from build123d import *

# Parameters (mm, degrees)
SCHIZZO1_R                        = 31.2
SCHIZZO1_R_2                      = 22.5
ESTRUSIONE_ESTRUSIONE1_DEPTH      = 40
SCHIZZO2_R                        = 2.25
TAGLIO_ESTRUSIONE1_DEPTH          = 60.555688225
RIPETIZIONECIRCOLARE1_COUNT       = 9
SCHIZZO3_W                        = 40
SCHIZZO3_H                        = 62.4
TAGLIO_ESTRUSIONE2_DEPTH          = 39
ESTRUSIONE_ESTRUSIONE2_START      = -10
ESTRUSIONE_ESTRUSIONE2_DEPTH      = 10
SCHIZZO5_R                        = 8.05
TAGLIO_ESTRUSIONE3_DEPTH          = 5
SCHIZZO6_R                        = 6.05
TAGLIO_ESTRUSIONE6_DEPTH          = 57.31944602
SCHIZZO7_R                        = 3.75
TAGLIO_ESTRUSIONE7_DEPTH          = 5
RIPETIZIONECIRCOLARE2_COUNT       = 9
ESTRUSIONE_ESTRUSIONE3_DEPTH      = 2
ESTRUSIONE_ESTRUSIONE3_DEPTH_BACK = 5
SMUSSO1_SIZE                      = 2
RACCORDO2_R                       = 4
ESTRUSIONE_ESTRUSIONE4_DEPTH      = 40
ESTRUSIONE_ESTRUSIONE5_START      = -10
ESTRUSIONE_ESTRUSIONE5_DEPTH      = 10


# Some blends are built 0.0001 mm under size
with BuildPart() as part:
    # Schizzo1 → Estrusione-Estrusione1 (new body)
    with BuildSketch(Plane.XY):
        Circle(SCHIZZO1_R)
        Circle(SCHIZZO1_R_2, mode=Mode.SUBTRACT)
    extrude(amount=ESTRUSIONE_ESTRUSIONE1_DEPTH)

    # Schizzo2 → Taglio-Estrusione1 (cut, through all)
    with BuildSketch(Plane.XY.offset(40)):
        with Locations((0, 27)):
            Circle(SCHIZZO2_R)
    taglio_estrusione1 = extrude(amount=-TAGLIO_ESTRUSIONE1_DEPTH, mode=Mode.SUBTRACT)

    # RipetizioneCircolare1: Taglio-Estrusione1 ×9 about axis
    ripetizionecircolare1_axis = Axis((0, 0, 0), (0, 0, 1))
    for i in range(1, RIPETIZIONECIRCOLARE1_COUNT):
        add(taglio_estrusione1.rotate(ripetizionecircolare1_axis, i * 360 / RIPETIZIONECIRCOLARE1_COUNT), mode=Mode.SUBTRACT)

    # Schizzo3 → Taglio-Estrusione2 (cut)
    with BuildSketch(Plane(origin=(0, 0, 0), x_dir=(0, 0, -1), z_dir=(1, 0, 0))):
        with Locations((-20, 0)):
            Rectangle(SCHIZZO3_W, SCHIZZO3_H)
    extrude(amount=-TAGLIO_ESTRUSIONE2_DEPTH, mode=Mode.SUBTRACT)

    # Schizzo4 → Estrusione-Estrusione2 (add)
    with BuildSketch(Plane.XY.offset(40).offset(ESTRUSIONE_ESTRUSIONE2_START)):
        with BuildLine():
            Line((0, 22.5), (0, -22.5))
            ThreePointArc((0, -22.5), (22.5, 0), (0, 22.5))
        make_face()
        with BuildLine():
            ThreePointArc((22.5, 0), (15.909902577, 15.909902577), (0, 22.5))
            Line((0, 22.5), (0, -22.5))
            ThreePointArc((0, -22.5), (15.909902577, -15.909902577), (22.5, 0))
        make_face()
        with BuildLine():
            Line((0, -22.5), (0, 22.5))
            ThreePointArc((0, 22.5), (-22.5, 0), (0, -22.5))
        make_face()
    extrude(amount=ESTRUSIONE_ESTRUSIONE2_DEPTH)

    # Schizzo5 → Taglio-Estrusione3 (cut)
    with BuildSketch(Plane.XY.offset(40)):
        Circle(SCHIZZO5_R)
    extrude(amount=-TAGLIO_ESTRUSIONE3_DEPTH, mode=Mode.SUBTRACT)

    # Schizzo6 → Taglio-Estrusione6 (cut, through all)
    with BuildSketch(Plane.XY.offset(35)):
        Circle(SCHIZZO6_R)
    extrude(amount=-TAGLIO_ESTRUSIONE6_DEPTH, mode=Mode.SUBTRACT)

    # Schizzo7 → Taglio-Estrusione7 (cut)
    with BuildSketch(Plane.XY.offset(40)):
        with Locations((17.355265462, 20.683199964)):
            Circle(SCHIZZO7_R)
    taglio_estrusione7 = extrude(amount=-TAGLIO_ESTRUSIONE7_DEPTH, mode=Mode.SUBTRACT)

    # RipetizioneCircolare2: Taglio-Estrusione7 ×9 about axis
    ripetizionecircolare2_axis = Axis((0, 0, 0), (0, 0, 1))
    for i in range(1, RIPETIZIONECIRCOLARE2_COUNT):
        add(taglio_estrusione7.rotate(ripetizionecircolare2_axis, i * 360 / RIPETIZIONECIRCOLARE2_COUNT), mode=Mode.SUBTRACT)

    # Schizzo8 → Estrusione-Estrusione3 (add, two sides: drawn at the far end of the back side and taken through both)
    with BuildSketch(Plane(origin=(0, 0, 0), x_dir=(-1, 0, 0), z_dir=(0, 0, -1)).offset(-ESTRUSIONE_ESTRUSIONE3_DEPTH_BACK)):
        with BuildLine():
            Line((0, 31.2), (0, 33.2))
            ThreePointArc((0, 33.2), (-33.2, 0), (0, -33.2))
            Line((0, -33.2), (0, -31.2))
            ThreePointArc((0, -31.2), (-31.2, 0), (0, 31.2))
        make_face()
    extrude(amount=ESTRUSIONE_ESTRUSIONE3_DEPTH + ESTRUSIONE_ESTRUSIONE3_DEPTH_BACK)

    # Smusso1
    smusso1_edges = [part.edges().sort_by_distance(p)[0] for p in [
        (31.2, 0, 5),
    ]]
    chamfer(smusso1_edges, length=SMUSSO1_SIZE - 0.0001)  # a hair under: the kernel refuses the full size

    # Raccordo2
    # the kernel refuses this fillet: 4 mm, written as the material it adds along each edge
    with BuildSketch(Plane(origin=(0, 0, 30), x_dir=(0, -1, 0), z_dir=(-1, 0, 0))) as raccordo2_piece_1:
        with BuildLine():
            CenterArc((22.5 - RACCORDO2_R, -RACCORDO2_R), RACCORDO2_R, 0, 90)
            Line((22.5 - RACCORDO2_R, 0), (22.5, 0))
            Line((22.5, 0), (22.5, -RACCORDO2_R))
        make_face()
    revolve(axis=Axis((0, 0, 30), (0, 0, 1)), revolution_arc=180)

    # Schizzo9 → Estrusione-Estrusione4 (add)
    with BuildSketch(Plane.XY.offset(40)):
        with BuildLine():
            Line((0, 30.75), (0, 23.25))
            ThreePointArc((0, 23.25), (3.75, 27), (0, 30.75))
        make_face()
    extrude(amount=-ESTRUSIONE_ESTRUSIONE4_DEPTH)

    # Schizzo10 → Estrusione-Estrusione5 (add)
    with BuildSketch(Plane.XY.offset(40).offset(ESTRUSIONE_ESTRUSIONE5_START)):
        with BuildLine():
            Line((0, 22.5), (0, 31.2))
            Line((0, 31.2), (-15.587436356, 16.225961538))
            ThreePointArc((-15.587436356, 16.225961538), (-8.40136493, 20.872639203), (0, 22.5))
        make_face()
        with BuildLine():
            ThreePointArc((0, -22.5), (-8.40136493, -20.872639203), (-15.587436356, -16.225961538))
            Line((-15.587436356, -16.225961538), (0, -31.2))
            Line((0, -31.2), (0, -22.5))
        make_face()
    extrude(amount=ESTRUSIONE_ESTRUSIONE5_DEPTH)


solid = part.part
The model under review builds one solid part; all positions refer to its coordinate system, in mm. A direction names the side the tool comes from. Give positions to 0.01 mm unless a question says otherwise; leave off trailing zeros. Write each loop counter-clockwise with the first axis right and the second up, starting at its lowest first coordinate (ties: lowest second). Pieces come first, ordered by that corner, then holes. Notation, with made-up numbers: M 12,66.5 L 21,66.5 A13 cw 21,79.5 Z; hole C -0.5,24.5 d5. An arc over 180 degrees is marked long. One line per question, with ' | ' between items. Start each with the question number.
Item 1: For faces 4 (the flat face through (0, 28, 14)), 5 (the cylindrical face through (23.61, 2.41, 37.53)), 6 (the cylindrical face through (24.342, 4.787, 17.745)), 7 (the flat face through (24, 0, 0)), list the 3-axis set-ups (+Z, -Z, +X, -X, +Y, -Y) from which the entire face can be reached by the end or side of a thin tool; tool diameter is ignored.
Item 2: Wall thickness on line 1 (Y direction, x = 18, z = 22); line 2 (X direction, y = 4, z = 27); line 3 (Y direction, x = 28, z = 21.5): over which ranges is each line inside the solid? List them lowest first. Write a range as from..to.
Item 3: We need section C-C on z = 34. Write out the cut boundary in (x, y), plus the area to 3 significant figures.
Item 4: We need section A-A on z = 10. Write out the cut boundary in (x, y).
Item 5: Draft analysis for pull direction Y (two halves, no side actions). For faces 1 (the cylindrical face through (31.192, -0.686, 23.269)), 2 (the flat face through (31.4, 0.2, -2)), 3 (the flat face through (-2, 6, 35)), state which applies: released by +Y, released by -Y, zero draft, split by the parting line, or undercut.
Item 6: For pin 1 (12 mm diameter, centred on y = -10.5, z = 29, fed in from +X); pin 2 (8 mm diameter, centred on x = 7, z = 23.5, fed in from +Y); pin 3 (2 mm diameter, centred on x = 18.5, y = 22, fed in from +Z), all flat-tipped, find the tip position at first contact; note any pin that passes through.
Results found:
1) face 4: -Z, -X, +Y, -Y | face 5: +Z | face 6: +Z, -Z | face 7: -Z, -X
2) line 1: y = -25.48..-13.5, 13.5..18.53, 22.84..25.48 | line 2: x = 22.01..24.45, 28.73..30.94 | line 3: y = -13.76..2.94, 6.44..13.76
3) outline: M -15.59,-16.23 L 0,-31.2 A31.2 ccw 0,31.2 L -15.59,16.23 A22.5 ccw Z; hole C 0,0 d12.1; hole C 9.23,-25.37 d4.5; hole C 17.36,20.68 d4.5; hole C 23.38,-13.5 d4.5; hole C 26.59,4.69 d4.5 | area: 2,240 mm2
4) outline: M 0,-31.2 A31.2 ccw 0,31.2 L 0,22.5 A22.5 cw 0,-22.5 Z; hole C 9.23,-25.37 d4.5; hole C 17.36,20.68 d4.5; hole C 23.38,-13.5 d4.5; hole C 26.59,4.69 d4.5
5) face 1: split by the parting line | face 2: zero draft | face 3: undercut
6) pin 1: stops at x = 30.87 | pin 2: stops at y = 31.06 | pin 3: stops at z = 35
